Can you work these out from the model? Positions are in its coordinate system, mm. A direction names the side the tool comes from. Coordinates: 2 decimals unless noted, no trailing zeros. Write each loop counter-clockwise with the first axis right and the second up, starting at its lowest first coordinate (ties: lowest second). Pieces come first, ordered by that corner, then holes. Notation, with made-up numbers: M 50,24.5 L 71,24.5 A22 ccw 71,35.5 Z; hole C 41,43 d5. An arc over 180 degrees is marked long. Answer as a JSON object with one key per item and string values. Group by question number.
from build123d import *

# Parameters (mm, degrees)
BASE_FLANGE1_DEPTH                              = 55
CUT_EXTRUDE2_REACH                              = 115.264
SKETCH6_R                                       = 10.5
CUT_EXTRUDE3_REACH                              = 115.888
SKETCH7_W                                       = 90.6
SKETCH7_H                                       = 68.2
CSK_FOR_M2_FLAT_HEAD_MACHINE_SCREW1_D           = 2.4
CSK_FOR_M2_FLAT_HEAD_MACHINE_SCREW1_CSINK_D     = 4.4
CSK_FOR_M2_FLAT_HEAD_MACHINE_SCREW1_CSINK_ANGLE = 90


# Sheet-metal steps are written as plain solids
with BuildPart() as part:
    # Sketch1 → Base-Flange1 (new, symmetric)
    with BuildSketch(Plane.XY):
        with BuildLine():
            Line((70, -30), (70, 68.545432303))
            ThreePointArc((70, 68.545432303), (69.784254855, 69.066287158), (69.2634, 69.282032303))
            Line((69.2634, 69.282032303), (40.425276208, 69.282032303))
            ThreePointArc((40.425276208, 69.282032303), (40.056976208, 69.183346615), (39.787361896, 68.913732303))
            Line((39.787361896, 68.913732303), (0.425276208, 0.7366))
            ThreePointArc((0.425276208, 0.7366), (-0.113952417, 0.197371375), (-0.850552417, 0))
            Line((-0.850552417, 0), (-59.2634, 0))
            ThreePointArc((-59.2634, 0), (-59.784254855, -0.215745145), (-60, -0.7366))
            Line((-60, -0.7366), (-60, -30))
            Line((-60, -30), (-60.7366, -30))
            Line((-60.7366, -30), (-60.7366, -0.7366))
            ThreePointArc((-60.7366, -0.7366), (-60.30510971, 0.30510971), (-59.2634, 0.7366))
            Line((-59.2634, 0.7366), (-0.850552417, 0.7366))
            ThreePointArc((-0.850552417, 0.7366), (-0.482252417, 0.835285688), (-0.212638104, 1.1049))
            Line((-0.212638104, 1.1049), (39.149447583, 69.282032303))
            ThreePointArc((39.149447583, 69.282032303), (39.688676208, 69.821260928), (40.425276208, 70.018632303))
            Line((40.425276208, 70.018632303), (69.2634, 70.018632303))
            ThreePointArc((69.2634, 70.018632303), (70.30510971, 69.587142013), (70.7366, 68.545432303))
            Line((70.7366, 68.545432303), (70.7366, -30))
            Line((70.7366, -30), (70, -30))
        make_face()
    extrude(amount=BASE_FLANGE1_DEPTH, both=True)

    # Sketch6 → Cut-Extrude2 (cut, up to next)
    with BuildSketch(Plane(origin=(0, 0.7366, 0), x_dir=(1, 0, 0), z_dir=(0, 1, 0)), mode=Mode.PRIVATE) as cut_extrude2_sk1:
        with Locations(Location((-39.2634, 14, 0), (0, 0, 180))):
            Circle(SKETCH6_R)
    cut_extrude2_tool1 = extrude(cut_extrude2_sk1.sketch, amount=-CUT_EXTRUDE2_REACH, mode=Mode.PRIVATE) & part.part
    # Sketch6 → Cut-Extrude2 (cut, up to next)
    with BuildSketch(Plane(origin=(0, 0.7366, 0), x_dir=(1, 0, 0), z_dir=(0, 1, 0)), mode=Mode.PRIVATE) as cut_extrude2_sk2:
        with Locations(Location((-39.2634, 37, 0), (0, 0, 180))):
            Circle(SKETCH6_R)
    cut_extrude2_tool2 = extrude(cut_extrude2_sk2.sketch, amount=-CUT_EXTRUDE2_REACH, mode=Mode.PRIVATE) & part.part
    # Sketch6 → Cut-Extrude2 (cut, up to next)
    with BuildSketch(Plane(origin=(0, 0.7366, 0), x_dir=(1, 0, 0), z_dir=(0, 1, 0)), mode=Mode.PRIVATE) as cut_extrude2_sk3:
        with Locations(Location((-39.2634, -14, 0), (0, 0, 180))):
            Circle(SKETCH6_R)
    cut_extrude2_tool3 = extrude(cut_extrude2_sk3.sketch, amount=-CUT_EXTRUDE2_REACH, mode=Mode.PRIVATE) & part.part
    # Sketch6 → Cut-Extrude2 (cut, up to next)
    with BuildSketch(Plane(origin=(0, 0.7366, 0), x_dir=(1, 0, 0), z_dir=(0, 1, 0)), mode=Mode.PRIVATE) as cut_extrude2_sk4:
        with Locations(Location((-39.2634, -37, 0), (0, 0, 180))):
            Circle(SKETCH6_R)
    cut_extrude2_tool4 = extrude(cut_extrude2_sk4.sketch, amount=-CUT_EXTRUDE2_REACH, mode=Mode.PRIVATE) & part.part
    add(cut_extrude2_tool1.solids().sort_by_distance((-39.2634, 0.7366, -14))[0], mode=Mode.SUBTRACT)
    add(cut_extrude2_tool2.solids().sort_by_distance((-39.2634, 0.7366, -37))[0], mode=Mode.SUBTRACT)
    add(cut_extrude2_tool3.solids().sort_by_distance((-39.2634, 0.7366, 14))[0], mode=Mode.SUBTRACT)
    add(cut_extrude2_tool4.solids().sort_by_distance((-39.2634, 0.7366, 37))[0], mode=Mode.SUBTRACT)

    # Sketch7 → Cut-Extrude3 (cut, up to next)
    with BuildSketch(Plane(origin=(-0.637914312, 0.3683, 0), x_dir=(0, 0, 1), z_dir=(-0.8660254037844365, 0.500000000000004, 0)), mode=Mode.PRIVATE) as cut_extrude3_sk1:
        with Locations((0, 42.174723792)):
            Rectangle(SKETCH7_W, SKETCH7_H)
    cut_extrude3_tool1 = extrude(cut_extrude3_sk1.sketch, amount=-CUT_EXTRUDE3_REACH, mode=Mode.PRIVATE) & part.part
    add(cut_extrude3_tool1.solids().sort_by_distance((20.449448, 36.892682, 0))[0], mode=Mode.SUBTRACT)

    # CSK for M2 Flat Head Machine Screw1 (through all)
    with Locations(Plane(origin=(0, 0.7366, 0), x_dir=(1, 0, 0), z_dir=(0, 1, 0))):
        with Locations((-53.2634, 47), (-11.2634, 47), (-11.2634, -47), (-53.2634, -47)):
            CounterSinkHole(CSK_FOR_M2_FLAT_HEAD_MACHINE_SCREW1_D / 2, CSK_FOR_M2_FLAT_HEAD_MACHINE_SCREW1_CSINK_D / 2, counter_sink_angle=CSK_FOR_M2_FLAT_HEAD_MACHINE_SCREW1_CSINK_ANGLE)


solid = part.part
Q1. If we section it at C-C on x = 6: List the corners of the cut face in (y, z) for me, and give its area (3 significant figures).
Q2. If we section it at D-D on x = -42.5: List the corners of the cut face in (y, z) for me.
Q3. If we section it at B-B on z = 14: List the corners of the cut face in (x, y) for me, and give its area (3 significant figures).
Q4. Please list where these lines run through material, in increasing order: L1, parallel to X at y = -7, z = 15.5; L2, parallel to Y at x = -21, z = 0; L3, parallel to X at y = 3, z = -46.
Q5. Will these pins go through, and if not, where does the flat tip stop? pin 1 (24 mm diameter, centred on x = -39.26, z = -37, fed in from +Y); pin 2 (10 mm diameter, centred on x = -29, y = -8.5, fed in from +Z); pin 3 (10.5 mm diameter, centred on x = 17.5, y = 41.5, fed in from +Z).
Q6. On a 3-axis mill with a long thin cutter (end or side, diameter ignored), from which of +Z, -Z, +X, -X, +Y, -Y can I reach the whole of each face in a straight line? I mean faces 1 (the flat face through (55, 69.282, 1)), 2 (the cylindrical face through (-48.963, 0.373, 32.978)). Say none if no direction works.
Q7. If we section it at A-A on y = -19: List the corners of the cut face in (x, z) for me, and give its area (3 significant figures).
Q8. We'd pull the mould along X, two halves only. Please class faces 3 (the flat face through (70.737, 20, 1)), 4 (the flat face through (-30, 0, 1)), 5 (the flat face through (20.5, 36.3, 45.3)): pulls with the +X half, pulls with the -X half, needs draft (parallel to the pull), parting line crosses it, or undercut.
Reply:
{
 "1": {"outline": "M 10.39,-55 L 11.87,-55 L 11.87,-45.3 L 10.39,-45.3 Z; M 10.39,45.3 L 11.87,45.3 L 11.87,55 L 10.39,55 Z", "area": "28.6 mm^2"},
 "2": {"outline": "M 0,-55 L 0.74,-55 L 0.74,-46.99 L 0,-46.99 Z; M 0,-27.01 L 0.74,-27.01 L 0.74,-23.99 L 0,-23.99 Z; M 0,-4.01 L 0.74,-4.01 L 0.74,4.01 L 0,4.01 Z; M 0,23.99 L 0.74,23.99 L 0.74,27.01 L 0,27.01 Z; M 0,46.99 L 0.74,46.99 L 0.74,55 L 0,55 Z"},
 "3": {"outline": "M -60.74,-30 L -60,-30 L -60,-0.74 A0.74 cw -59.26,0 L -49.76,0 L -49.76,0.74 L -59.26,0.74 A1.47 ccw -60.74,-0.74 Z; M -28.76,0 L -0.85,0 A1.47 ccw 0.43,0.74 L 4.04,6.99 L 3.4,7.36 L -0.21,1.1 A0.74 cw -0.85,0.74 L -28.76,0.74 Z; M 37.5,66.42 L 38.14,66.06 L 39.79,68.91 A0.74 cw 40.43,69.28 L 69.26,69.28 A0.74 cw 70,68.55 L 70,-30 L 70.74,-30 L 70.74,68.55 A1.47 ccw 69.26,70.02 L 40.43,70.02 A1.47 ccw 39.15,69.28 Z", "area": "155 mm^2"},
 "4": {"L1": "-60.74 to -60, 70 to 70.74", "L2": "0 to 0.74", "L3": "0.88 to 1.73, 70 to 70.74"},
 "5": {"pin 1": "y = 0.74", "pin 2": "through", "pin 3": "z = 55"},
 "6": {"face 1": "+Z, -Z, -Y", "face 2": "+Y, -Y"},
 "7": {"outline": "M -60.74,-55 L -60,-55 L -60,55 L -60.74,55 Z; M 70,-55 L 70.74,-55 L 70.74,55 L 70,55 Z", "area": "162 mm^2"},
 "8": {"face 3": "pulls with the +X half", "face 4": "undercut", "face 5": "needs draft"}
}
